For this review, take the finished solid that the model builds, in its own axes (mm). A direction names the side the tool comes from. Coordinates: 2 decimals unless noted, no trailing zeros. Write each loop counter-clockwise with the first axis right and the second up, starting at its lowest first coordinate (ties: lowest second). Pieces come first, ordered by that corner, then holes. Notation, with made-up numbers: M 28,24.25 L 84,24.25 A11 ccw 84,34.25 Z; hole C -38.75,51.5 d4. An arc over 180 degrees is marked long. One line per question, with ' | ' between items.
from build123d import *

# Parameters (mm, degrees)
SKETCH1_W           = 75
SKETCH1_H           = 126.51894577
SKETCH1_R           = 1.875
SKETCH1_R_2         = 1.765
BOSS_EXTRUDE2_DEPTH = 2


with BuildPart() as part:
    # Sketch1 → Boss-Extrude2 (new body)
    with BuildSketch(Plane.XY):
        with Locations((0, -201.288893998)):
            Rectangle(SKETCH1_W, SKETCH1_H)
        with Locations((32.5, -259.548366883)):
            Circle(SKETCH1_R, mode=Mode.SUBTRACT)
        with Locations((-32.5, -259.548366883)):
            Circle(SKETCH1_R, mode=Mode.SUBTRACT)
        with Locations((-32.5, -194.548366883)):
            Circle(SKETCH1_R, mode=Mode.SUBTRACT)
        with Locations((32.5, -194.548366883)):
            Circle(SKETCH1_R, mode=Mode.SUBTRACT)
        with Locations((14.329505719, -159.529421113)):
            Circle(SKETCH1_R_2, mode=Mode.SUBTRACT)
        with Locations((-14.329505719, -159.529421113)):
            Circle(SKETCH1_R_2, mode=Mode.SUBTRACT)
        Polygon((-27.5, -204.548366883), (-27.5, -249.548366883), (-5, -227.048366883), align=None, mode=Mode.SUBTRACT)
        Polygon((-22.5, -254.548366883), (22.5, -254.548366883), (0, -232.048366883), align=None, mode=Mode.SUBTRACT)
        Polygon((27.5, -249.548366883), (27.5, -204.548366883), (5, -227.048366883), align=None, mode=Mode.SUBTRACT)
        Polygon((-22.5, -199.548366883), (22.5, -199.548366883), (0, -222.048366883), align=None, mode=Mode.SUBTRACT)
        Polygon((-22.5, -189.548366883), (22.5, -189.548366883), (0, -167.048366883), align=None, mode=Mode.SUBTRACT)
        Polygon((14.024331064, -145.954035819), (0, -159.978366883), (-13.95827912, -146.020087763), align=None, mode=Mode.SUBTRACT)
    extrude(amount=BOSS_EXTRUDE2_DEPTH)


solid = part.part
1. Take a section at D-D on y = -176. State the section outline as (x, z) points, plus the area to 3 significant figures.
Computed values:
outline: M -37.5,0 L -8.95,0 L -8.95,2 L -37.5,2 Z; M 8.95,0 L 37.5,0 L 37.5,2 L 8.95,2 Z | area: 114 mm2
2. Take a section at A-A on x = -32.5. State the section outline as (y, z) points, plus the area to 3 significant figures.
Computed values:
outline: M -264.55,0 L -261.42,0 L -261.42,2 L -264.55,2 Z; M -257.67,0 L -196.42,0 L -196.42,2 L -257.67,2 Z; M -192.67,0 L -138.03,0 L -138.03,2 L -192.67,2 Z | area: 238 mm2
3. Take a section at B-B on x = 9. State the section outline as (y, z) points.
Computed values:
outline: M -264.55,0 L -254.55,0 L -254.55,2 L -264.55,2 Z; M -241.05,0 L -231.05,0 L -231.05,2 L -241.05,2 Z; M -223.05,0 L -213.05,0 L -213.05,2 L -223.05,2 Z; M -199.55,0 L -189.55,0 L -189.55,2 L -199.55,2 Z; M -176.05,0 L -150.98,0 L -150.98,2 L -176.05,2 Z; M -145.97,0 L -138.03,0 L -138.03,2 L -145.97,2 Z
4. Draft analysis for pull direction X (two halves, no side actions). For faces 3 (the flat face through (7.8, -214.5, 0)), 4 (the cylindrical face through (33.37, -261.21, 0.99)), state which applies: pulls with the +X half, pulls with the -X half, needs draft (parallel to the pull), parting line crosses it, or undercut.
Computed values:
face 3: needs draft | face 4: undercut
5. Take a section at C-C on z = 0.9. Give the number of separate pieces and of enclosed holes in the cut face, plus the area to 3 significant figures.
Computed values:
separate pieces: 1 | enclosed holes: 12 | area: 6,700 mm2
6. Clearance check with a flat-ended pin moving along its axis: P1, Ø5, axis at x = -32.5, y = -194.55, coming from the +Z side. State where the tip first meets the part, or that it passes through.
Computed values:
P1: stops at z = 2
7. Machinability: for faces 1 (the flat face through (7.8, -214.5, 2)), 2 (the flat face through (16.09, -238.14, 0.99)), which of the approach directions +Z, -Z, +X, -X, +Y, -Y give a long, thin tool a straight path to every point of the face, cutting with its end or side? Answer none if there is none.
Computed values:
face 1: +Z, +X, -X, +Y, -Y | face 2: +Z, -Z
8. For line 1 along Y through (x, z) = (-32.5, 0.85); line 2 along Y through (x, z) = (-11, 0.2); line 3 along X through (y, z) = (-239, 0.75), list the stretches that pass through material, from the lowest coordinate up.
Computed values:
line 1: y = -264.55 to -261.42, -257.67 to -196.42, -192.67 to -138.03 | line 2: y = -264.55 to -254.55, -243.05 to -233.05, -221.05 to -211.05, -199.55 to -189.55, -178.05 to -148.98, -146.01 to -138.03 | line 3: x = -37.5 to -27.5, -16.95 to -6.95, 6.95 to 16.95, 27.5 to 37.5
